```python
from build123d import *

# Parameters (mm, degrees)
SKETCH_2_R          = 12
SKETCH_2_R_2        = 5
CUT_EXTRUDE_1_DEPTH = 3
SKETCH_3_W          = 5
SKETCH_3_H          = 2


with BuildPart() as part:
    # 草图1 → 旋转1 (revolve)
    with BuildSketch(Plane(origin=(0, 0, 0), x_dir=(0, 0, -1), z_dir=(1, 0, 0))):
        with BuildLine():
            Line((-76, 5), (-20, 5))
            Line((-20, 5), (-11, 14))
            Line((-11, 14), (-8, 14))
            Line((-8, 14), (-8, 5))
            Line((-8, 5), (0, 5))
            Line((0, 5), (0, 0))
            Line((0, 0), (-81, 0))
            ThreePointArc((-81, 0), (-79.535533906, 3.535533906), (-76, 5))
        make_face()
    revolve(axis=Axis((0, 0, 0), (0, 0, 1)))

    # 草图2 → 切除-拉伸1 (cut)
    with BuildSketch(Plane(origin=(0, 0, 8), x_dir=(-1, 0, 0), z_dir=(0, 0, -1))):
        with Locations(Location((0, 0, 0), (0, 0, 90))):
            Circle(SKETCH_2_R)
        with Locations(Location((0, 0, 0), (0, 0, 90))):
            Circle(SKETCH_2_R_2, mode=Mode.SUBTRACT)
    extrude(amount=-CUT_EXTRUDE_1_DEPTH, mode=Mode.SUBTRACT)

    # 草图3 → 切除-旋转1 (revolve, cut)
    with BuildSketch(Plane(origin=(0, 0, 0), x_dir=(1, 0, 0), z_dir=(0, 1, 0)), mode=Mode.PRIVATE) as cut_revolve_1_sk:
        with Locations((7.5, -19)):
            Rectangle(SKETCH_3_W, SKETCH_3_H)
    revolve(cut_revolve_1_sk.sketch.rotate(Axis((0, 0, 20), (0, 0, 1)), 90), axis=Axis((0, 0, 20), (0, 0, 1)), mode=Mode.SUBTRACT)


solid = part.part
```
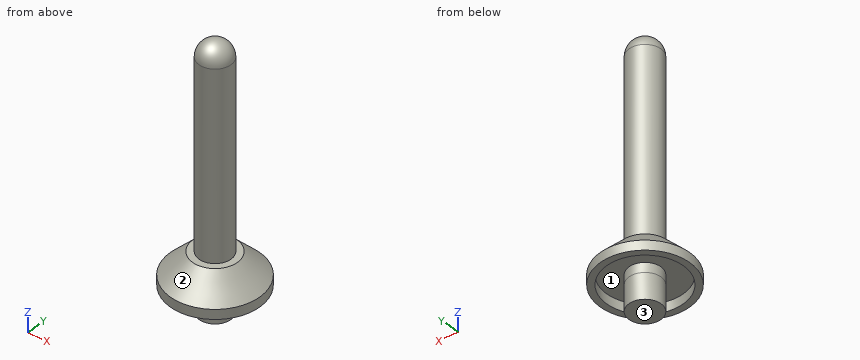
Model file for the job. Use its own axes, mm. Face numbers are marked on the shaded views. Round coordinates to 2 decimals unless told otherwise and drop trailing zeros. Write each loop counter-clockwise with the first axis right and the second up, starting at its lowest first coordinate (ties: lowest second). Pieces come first, ordered by that corner, then holes. Notation, with made-up numbers: (19, 8) -> (42, 8) arc R14 ccw to (42, 33) -> close; hole circle Ø6 at (86, -32.5). An arc over 180 degrees is marked (long way). Answer as CSV lines item,"result".
1. Mould opens along Y. For the marked faces 1, 2 and 3 say: +Y half, -Y half, draft (parallel to the pull), parting line (faces both ways), or undercut.
Resolved:
face 1,"undercut"
face 2,"parting line"
face 3,"draft"
2. Slice it at A-A, the plane x = 0. List the corners of the cut face in (y, z).
Resolved:
outline,"(-14, 8) -> (-12, 8) -> (-12, 11) -> (-5, 11) -> (-5, 0) -> (5, 0) -> (5, 11) -> (12, 11) -> (12, 8) -> (14, 8) -> (14, 11) -> (7, 18) -> (5, 18) -> (5, 76) arc R5 ccw to (-5, 76) -> (-5, 18) -> (-7, 18) -> (-14, 11) -> close"
3. Slice it at C-C, the plane z = 38. List the corners of the cut face in (x, y).
Resolved:
outline,"circle Ø10 at (0, 0)"
4. Drill centre lines: line 1 (X direction, y = 0, z = 8.7); line 2 (Y direction, x = -0.25, z = 51); line 3 (Z direction, x = -7.75, y = -2.5). Where is each one in solid material? Low to high.
Resolved:
line 1,"-14 to -12, -5 to 5, 12 to 14"
line 2,"-4.99 to 4.99"
line 3,"11 to 16.86"
5. Pin check, flat tips, straight feed: pin 1 Ø4 at (x, y) = (2, -1.5) entering from +Z; pin 2 Ø6 at (y, z) = (-3, 70) entering from +X; pin 3 Ø3 at (x, z) = (-4, 26) entering from -Y. Stop position of each tip, or through.
Resolved:
pin 1,"z = 80.97"
pin 2,"x = 5"
pin 3,"y = -4.33"
